The model under review builds one solid part; all positions refer to its coordinate system, in mm. Give positions to 0.01 mm unless a question says otherwise; leave off trailing zeros. Loops run counter-clockwise (first coordinate to the right, second up) from the corner with the lowest first, then second, coordinate; pieces in that order, holes last. Notation, with made-up numbers: (10.5, 5.25) - (28.5, 5.25) arc R14 cw to (28.5, 19.25) - close; hole circle Ø10 at (52.5, 81). An arc over 180 degrees is marked (long way). Return JSON: item names as keys, results as strings. Group by question number.
```python
from build123d import *

# Parameters (mm, degrees)
SKETCH1_W                  = 116
SKETCH1_H                  = 90
BOSS_EXTRUDE1_DEPTH        = 1.6
F_3_5_3_5_DIAMETER_HOLE1_D = 3.5
FILLET1_R                  = 5
F_2_8_2_8_DIAMETER_HOLE1_D = 2.8


with BuildPart() as part:
    # Sketch1 → Boss-Extrude1 (new body)
    with BuildSketch(Plane.XY):
        with Locations((-39, 41)):
            Rectangle(SKETCH1_W, SKETCH1_H)
    extrude(amount=BOSS_EXTRUDE1_DEPTH)

    # Ø3.5 (3.5) Diameter Hole1 (through all)
    with Locations(Plane.XY.offset(1.6)):
        with Locations((0, 0), (15, 82), (-93, 82), (-93, 22)):
            Hole(F_3_5_3_5_DIAMETER_HOLE1_D / 2)

    # Fillet1
    fillet1_edges = [part.edges().sort_by_distance(p)[0] for p in [
        (-97, 86, 0.8),
        (19, 86, 0.8),
        (19, -4, 0.8),
        (-97, -4, 0.8),
    ]]
    fillet(fillet1_edges, radius=FILLET1_R)

    # Ø2.8 (2.8) Diameter Hole1 (through all)
    with Locations(Plane(origin=(0, 0, 0), x_dir=(-1, 0, 0), z_dir=(0, 0, -1))):
        with Locations((34.5, 75.1), (83.5, 75.1), (83.5, 17.1), (34.5, 17.1)):
            Hole(F_2_8_2_8_DIAMETER_HOLE1_D / 2)


solid = part.part
```
1) For pin 1 Ø2 at (x, y) = (-93, 82) entering from +Z, flat-tipped, find the tip position at first contact; note if it passes through.
2) Draft analysis for pull direction Y (two halves, no side actions). For faces 1 (the face through (-96, -2, 1)), 2 (the face through (-92.62, 80.29, 0.79)), 3 (the face through (17, 85, 1)), state which applies: +Y half, -Y half, draft (parallel to the pull), parting line (faces both ways), or undercut.
3) We need section A-A, the plane y = 22. Write out the cut boundary in (x, z).
4) To check wall thickness, follow line 1 (X direction, y = 75.1, z = 1.15); line 2 (Y direction, x = -93, z = 0.5); line 3 (Y direction, x = -83, z = 1.3). State the ranges of each line that lie inside material, in increasing order.
Findings:
{
 "1": {"pin 1": "passes through"},
 "2": {"face 1": "-Y half", "face 2": "undercut", "face 3": "+Y half"},
 "3": {"outline": "(-97, 0) - (-94.75, 0) - (-94.75, 1.6) - (-97, 1.6) - close; (-91.25, 0) - (19, 0) - (19, 1.6) - (-91.25, 1.6) - close"},
 "4": {"line 1": "x = -97 to -84.9, -82.1 to -35.9, -33.1 to 19", "line 2": "y = -3.9 to 20.25, 23.75 to 80.25, 83.75 to 85.9", "line 3": "y = -4 to 15.79, 18.41 to 73.79, 76.41 to 86"}
}
